Read the model definition and answer for the solid it produces. Units are mm, in the model's axes. Coordinates: 2 decimals unless noted, no trailing zeros. One line per item, written item: value. Start each with the question number.
1. Find section A-A, the plane z = 123.5. State how many separate pieces and enclosed holes the cut face has, and give its area (3 significant figures).
2. Given P1, Ø1.6, axis at y = 2, z = 319.5, coming from the -X side; P2, Ø5, axis at y = -0.5, z = -23.5, coming from the -X side; P3, Ø2, axis at y = -1, z = -117.5, coming from the +X side, each flat-ended and moving along its own axis, determine where each tip first touches the part or whether it passes through.
3. For a pull along X with two mould halves and no side action, classify faces 1 (the flat face through (-5.864, -0.07, 62.161)), 2 (the flat face through (-2.476, -0.07, 72.549)), 3 (the flat face through (-3.718, -0.07, 59.808)), 4 (the flat face through (-1, 5, 66)) as pulls with the +X half, pulls with the -X half, needs draft (parallel to the pull), parting line crosses it, or undercut.
```python
from build123d import *

# Parameters (mm, degrees)
F1_DEPTH = 5
F3_W     = 10
F3_H     = 10
F4_DEPTH = 2
F5_R     = 0.5


with BuildPart() as f1:
    # F0 (on Front) → F1 (new body, symmetric)
    with BuildSketch(Plane.XZ):
        Polygon((249.854166, 313.379943), (249.854166, 318.379943), (-250.145834, 318.379943), (-250.145834, 313.379943), (238.354166, 313.379943), (239.354166, 313.379943), (239.854166, 313.379943), (240.854166, 313.379943), (241.354166, 313.379943), (242.354166, 313.379943), (242.854166, 313.379943), (243.854166, 313.379943), (244.354166, 313.379943), (245.354166, 313.379943), (245.854166, 313.379943), (246.854166, 313.379943), (247.354166, 313.379943), (248.354166, 313.379943), (248.854166, 313.379943), align=None)
        Polygon((-250.145834, -185.120057), (248.354166, 313.379943), (247.354166, 313.379943), (-250.145834, -184.120057), align=None)
        Polygon((-250.145834, -186.620057), (249.854166, 313.379943), (248.854166, 313.379943), (-250.145834, -185.620057), align=None)
        Polygon((-250.145834, -182.120057), (245.354166, 313.379943), (244.354166, 313.379943), (-250.145834, -181.120057), align=None)
        Polygon((-250.145834, -183.620057), (246.854166, 313.379943), (245.854166, 313.379943), (-250.145834, -182.620057), align=None)
        Polygon((240.854166, 313.379943), (239.854166, 313.379943), (-250.145834, -176.620057), (-250.145834, -177.620057), align=None)
        Polygon((242.354166, 313.379943), (241.354166, 313.379943), (-250.145834, -178.120057), (-250.145834, -179.120057), align=None)
        Polygon((-250.145834, -180.620057), (243.854166, 313.379943), (242.854166, 313.379943), (-250.145834, -179.620057), align=None)
        Polygon((239.354166, 313.379943), (238.354166, 313.379943), (-250.145834, -175.120057), (-250.145834, -176.120057), align=None)
    extrude(amount=F1_DEPTH, both=True)

    # F3 (on face) → F4 (join)
    with BuildSketch(Plane.XY.offset(318.379943)):
        with Locations((244.854166, 0)):
            Rectangle(F3_W, F3_H)
    extrude(amount=F4_DEPTH)

    # F5
    f5_edges = [f1.edges().sort_by_distance(p)[0] for p in [
        (239.854166, 0, 318.379943),
        (249.854166, 0, 313.379943),
    ]]
    fillet(f5_edges, radius=F5_R)


solid = f1.part
```
Answer block:
1. separate pieces: 8
1. enclosed holes: 0
1. area: 80.0 mm2
2. P1: stops at x = 239.82
2. P2: stops at x = -101.03
2. P3: stops at x = -180.03
3. face 1: undercut
3. face 2: pulls with the -X half
3. face 3: pulls with the +X half
3. face 4: needs draft
